Input: dimensioned drawing with shaded views. Units: mm. Origin: part minimum x, y, z. Coordinates: 2 decimals unless noted, no trailing zeros. Loops run counter-clockwise (first coordinate to the right, second up) from the corner with the lowest first, then second, coordinate; pieces in that order, holes last. Notation, with made-up numbers: (86.5, -17.75) - (94.5, -17.75) arc R17 cw to (94.5, 2.25) - close; hole circle Ø1 at (2.5, -7). An arc over 180 degrees is marked (long way). Write item = value, one per line. Start each with the question number.
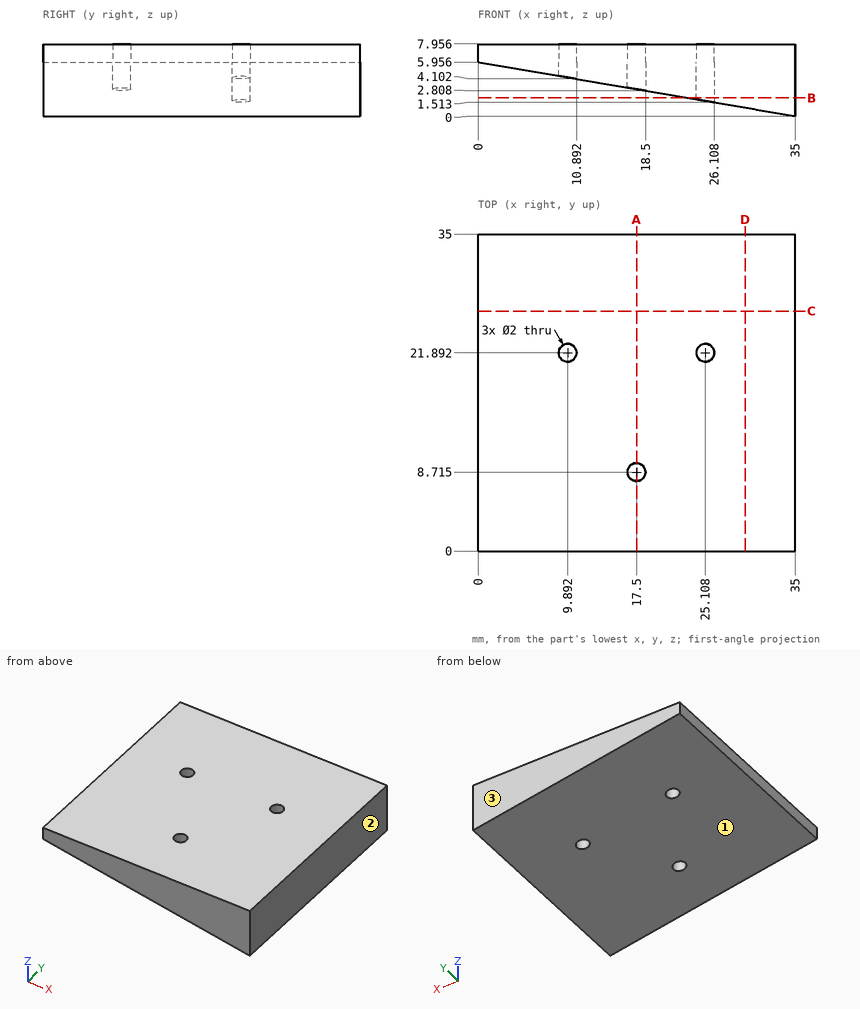
Item 1: Ray query, line 1 (Y direction, x = 18, z = 4.25); line 2 (Z direction, x = 18.5, y = 16.5) (1 decimal); line 3 (Z direction, x = 21.5, y = 23) (1 decimal). Return the intervals inside material, ascending.
Item 2: Pull-direction query (X, two-part tool) for the marked faces 1, 2 and 3; classes: pulls with the +X half, pulls with the -X half, needs draft (parallel to the pull), parting line crosses it, or undercut.
Item 3: Cut plane A-A on x = 17.5. Return loops of the section in (y, z) (1 decimal), plus the area to 3 significant figures.
Item 4: Cut plane C-C on y = 26.5. Return loops of the section in (x, z) (1 decimal).
Item 5: Pin query (flat end, axial travel): pin 1 (2.5 mm diameter, centred on x = 17.5, y = 8.715, fed in from -Z) (1 decimal); pin 2 (1 mm diameter, centred on x = 8, y = 4.5, fed in from -Z); pin 3 (2 mm diameter, centred on x = 8, y = 25.5, fed in from -Z). Return the tip coordinate at first contact, or that it passes through.
Item 6: Cut plane D-D on x = 29.5. Return loops of the section in (y, z) (1 decimal).
Item 7: Cut plane B-B on z = 2. Return loops of the section in (x, y).
Recorded:
q1.line_1 = 0 to 7.85, 9.58 to 35
q1.line_2 = 2.8 to 8
q1.line_3 = 2.3 to 8
q2.face_1 = pulls with the -X half
q2.face_2 = pulls with the +X half
q2.face_3 = needs draft
q3.outline = (0, 3) - (7.7, 3) - (7.7, 8) - (0, 8) - close; (9.7, 3) - (35, 3) - (35, 8) - (9.7, 8) - close
q3.area = 164 mm²
q4.outline = (0, 6) - (35, 0) - (35, 8) - (0, 8) - close
q5.pin_1 = 2.8
q5.pin_2 = 4.51
q5.pin_3 = 4.42
q6.outline = (0, 0.9) - (35, 0.9) - (35, 8) - (0, 8) - close
q7.outline = (23.25, 0) - (35, 0) - (35, 35) - (23.25, 35) - close; hole circle Ø2 at (25.11, 21.89)
